Print and shaded views of the part. All mm, measured from the part's lowest x, y and z. Give positions to 0.01 mm unless a question says otherwise; leave off trailing zeros. Order: outer loops, then holes, each group sorted by start corner. A loop starts at its lowest first (then second) coordinate and runs counter-clockwise, first axis right, second up. Notation, with made-up numbers: (8, 65) -> (51, 65) arc R23 ccw to (51, 101) -> close; hole circle Ø3 at (74.5, 73). An arc over 180 degrees is marked (long way). One line per question, with ' | ' between items. Start each with the question number.
(1) Pin check, flat tip, straight feed: pin 1 Ø10 at (x, y) = (48, 169.5) entering from -Z. Stop position of the tip, or through.
(2) Cut at A-A (z = 26). Give the cut face in (x, y), then the cut area to 3 significant figures.
(3) Cut at B-B (y = 170). Give the cut face in (x, z).
(4) Drill centre lines: L1, parallel to Y at x = 50, z = 48; L2, parallel to X at y = 300, z = 43.5. Where is each one in solid material? Low to high. Write a range as from..to.
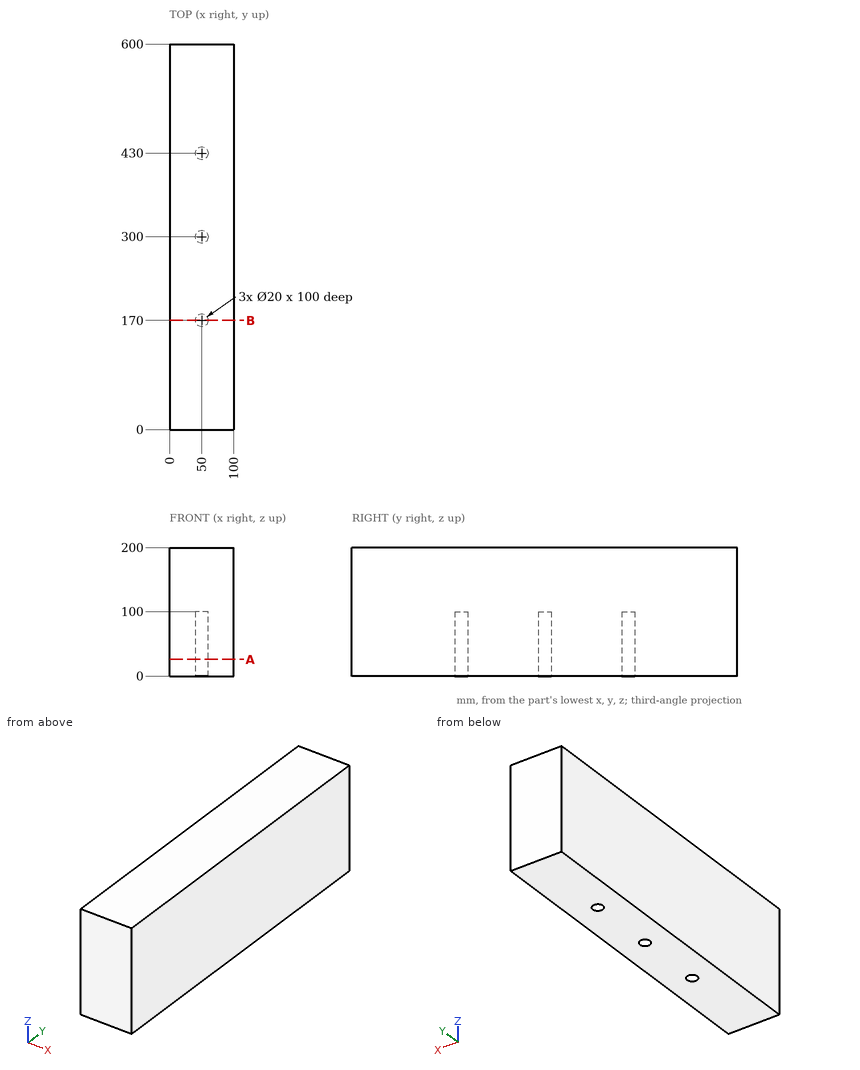
Result set:
1) pin 1: stops at z = 100
2) outline: (0, 0) -> (100, 0) -> (100, 600) -> (0, 600) -> close; hole circle Ø20 at (50, 170); hole circle Ø20 at (50, 300); hole circle Ø20 at (50, 430) | area: 59,100 mm2
3) outline: (0, 0) -> (40, 0) -> (40, 100) -> (60, 100) -> (60, 0) -> (100, 0) -> (100, 200) -> (0, 200) -> close
4) L1: y = 0..160, 180..290, 310..420, 440..600 | L2: x = 0..40, 60..100
